from build123d import *

# Parameters (mm, degrees)
F1_DEPTH  = 20
F3_DEPTH  = 10
F5_DEPTH  = 20
F6_R      = 10
F6_R_2    = 9.99999
F8_D      = 10
F10_D     = 10
F10_DEPTH = 10.001


# Not quite as in the source:
# - a fillet or chamfer is up to 0.001 mm smaller than in the source, because OpenCascade refuses the exact size


with BuildPart() as f1:
    # F0 (on Right) → F1 (new body, symmetric)
    with BuildSketch(Plane.YZ):
        Polygon((-60, 0), (0, 0), (0, 50), (-10, 50), (-10, 10), (-60, 10), align=None)
    extrude(amount=F1_DEPTH, both=True)

    # F2 (on Right) → F3 (join, symmetric)
    with BuildSketch(Plane.YZ):
        with BuildLine():
            Line((-60, 10), (-10, 10))
            Line((-10, 10), (-10, 30))
            Line((-10, 30), (-20, 30))
            Line((-20, 30), (-20, 40))
            ThreePointArc((-20, 40), (-22.9289321881, 47.0710678119), (-30, 50))
            Line((-30, 50), (-60, 50))
            Line((-60, 50), (-60, 10))
        make_face()
    extrude(amount=F3_DEPTH, both=True)

    # F4 (on face) → F5 (cut, through all)
    with BuildSketch(Plane.YZ.offset(10)):
        with BuildLine():
            Line((-60, 30), (-60, 10))
            Line((-60, 10), (-40, 10))
            ThreePointArc((-40, 10), (-30, 20), (-40, 30))
            Line((-40, 30), (-60, 30))
        make_face()
    extrude(amount=-F5_DEPTH, mode=Mode.SUBTRACT)

    # F6 (call 1 of 6: OpenCascade refuses the feature's edges together)
    f6_edges = [f1.edges().sort_by_distance(p)[0] for p in [
        (-20, -5, 50),
    ]]
    fillet(f6_edges, radius=F6_R)

    # F6#2 (call 2 of 6)
    f6_2_edges = [f1.edges().sort_by_distance(p)[0] for p in [
        (20, -5, 50),
    ]]
    fillet(f6_2_edges, radius=F6_R)

    # F6#3 (call 3 of 6)
    f6_3_edges = [f1.edges().sort_by_distance(p)[0] for p in [
        (-10, -60, 40),
    ]]
    fillet(f6_3_edges, radius=F6_R)

    # F6#4 (call 4 of 6) (radius 10 in the source; OpenCascade refuses exactly that, so slightly less here)
    f6_4_edges = [f1.edges().sort_by_distance(p)[0] for p in [
        (10, -60, 40),
    ]]
    fillet(f6_4_edges, radius=F6_R_2)

    # F6#5 (call 5 of 6) (radius 10 in the source; OpenCascade refuses exactly that, so slightly less here)
    f6_5_edges = [f1.edges().sort_by_distance(p)[0] for p in [
        (10, -10, 20),
    ]]
    fillet(f6_5_edges, radius=F6_R_2)

    # F6#6 (call 6 of 6) (radius 10 in the source; OpenCascade refuses exactly that, so slightly less here)
    f6_6_edges = [f1.edges().sort_by_distance(p)[0] for p in [
        (-10, -10, 20),
    ]]
    fillet(f6_6_edges, radius=F6_R_2)

    # F8 (through all)
    with Locations(Plane.XY.offset(50)):
        with Locations((0, -50)):
            Hole(F8_D / 2)

    # F10 (through all, one way)
    with BuildSketch(Plane.XZ.offset(10)):
        with Locations((-10, 40), (10, 40)):
            Circle(F10_D / 2)
    extrude(amount=-F10_DEPTH, mode=Mode.SUBTRACT)


solid = f1.part
Model file for the job. Use its own axes, mm. A direction names the side the tool comes from. Coordinates: 2 decimals unless noted, no trailing zeros. Order: outer loops, then holes, each group sorted by start corner. A loop starts at its lowest first (then second) coordinate and runs counter-clockwise, first axis right, second up. Notation, with made-up numbers: (50, 46) -> (90, 46) arc R21 cw to (90, 85) -> close; hole circle Ø3 at (26, 80.25). An arc over 180 degrees is marked (long way). Return JSON: item names as keys, results as strings. Group by question number.
Item 1: Pull direction Y, two halves, no side cores. Call faces 1 (the cylindrical face through (16.99, -5.07, 47.15)), 2 (the flat face through (0, -10, 39)), 3 (the cylindrical face through (-12.85, -13.01, 20.14)): pulls with the +Y half, pulls with the -Y half, needs draft (parallel to the pull), parting line crosses it, or undercut.
Item 2: Saw through at A-A on z = 46. State how many separate pieces and enclosed holes the cut face has, then the cut area to 3 significant figures.
Item 3: Saw through at D-D on z = 8.5. Write the cut outline in (x, y), then the cut area to 3 significant figures.
Item 4: Saw through at C-C on x = 8. Write the cut outline in (y, z), then the cut area to 3 significant figures.
Item 5: Wall check: line 1 along Z through (x, y) = (-8, -54.5); line 2 along Y through (x, z) = (0, 3.25); line 3 along Y through (x, z) = (1.5, 32). Give the ranges that are in metal, low to high. Write a range as [from, to].
Item 6: Tool access for faces 4 (the flat face through (10, -32, 35)), 5 (the cylindrical face through (-7.15, -56.99, 39.86)), 6 (the cylindrical face through (13, -5, 44)), 7 (the flat face through (0, -60, 5)), 8 (the flat face through (0, -20, 35)): list every direction of +Z, -Z, +X, -X, +Y, -Y with a clear straight run to the whole face (end or side of a thin tool).
Item 7: Saw through at B-B on y = -41.5. Write the cut outline in (x, z).
Item 8: Flat gauge pins, fed straight in: P1, Ø8, axis at x = 10, z = 40, coming from the +Y side; P2, Ø1, axis at x = -14, z = 16.5, coming from the -Y side; P3, Ø11, axis at x = 7, y = -16, coming from the +Z side. Where does each tip first touch, or does it go through?
Values found:
{
 "1": {"face 1": "needs draft", "face 2": "undercut", "face 3": "pulls with the -Y half"},
 "2": {"separate pieces": "2", "enclosed holes": "1", "area": "999 mm2"},
 "3": {"outline": "(-20, -60) -> (20, -60) -> (20, 0) -> (-20, 0) -> close; hole circle Ø10 at (0, -50)", "area": "2,320 mm2"},
 "4": {"outline": "(-60, 0) -> (0, 0) -> (0, 35.42) -> (-10, 35.42) -> (-10, 30) -> (-20, 30) -> (-20, 40) arc R10 ccw to (-30, 50) -> (-56, 50) -> (-56, 30) -> (-40, 30) arc R10 cw to (-40, 10) -> (-60, 10) -> close; (-10, 44.58) -> (0, 44.58) -> (0, 50) -> (-10, 50) -> close", "area": "2,050 mm2"},
 "5": {"line 1": "z = [0, 10], [30, 50]", "line 2": "y = [-60, -55], [-45, 0]", "line 3": "y = [-59.89, -54.77], [-45.23, -20], [-10, 0]"},
 "6": {"face 4": "+Z, +X, -Y", "face 5": "+Z, -X, -Y", "face 6": "+Y", "face 7": "+Z, -Z, +X, -X, -Y", "face 8": "+Z, +X, -X"},
 "7": {"outline": "(-20, 0) -> (20, 0) -> (20, 10) -> (-20, 10) -> close; (-10, 30) -> (10, 30) -> (10, 50) -> (-10, 50) -> close"},
 "8": {"P1": "stops at y = -20", "P2": "stops at y = -12.4", "P3": "stops at z = 45.27"}
}
